```python
from build123d import *

# Parameters (mm, degrees)
BOSS_EXTRUDE1_DEPTH = 6


with BuildPart() as part:
    # Sketch1 → Boss-Extrude1 (new body)
    with BuildSketch(Plane.XY.offset(6)):
        Polygon((302.766666667, 244), (302.766666667, 250), (282.033333333, 250), (282.033333333, 244), (260.3, 244), (260.3, 250), (239.566666667, 250), (239.566666667, 244), (217.833333333, 244), (217.833333333, 250), (197.1, 250), (197.1, 244), (175.366666667, 244), (175.366666667, 250), (154.633333333, 250), (154.633333333, 244), (132.9, 244), (132.9, 250), (112.166666667, 250), (112.166666667, 244), (90.433333333, 244), (90.433333333, 250), (69.7, 250), (69.7, 244), (47.966666667, 244), (47.966666667, 250), (27.233333333, 250), (27.233333333, 244), (6, 244), (6, 227.227272727), (0, 227.227272727), (0, 204.954545455), (6, 204.954545455), (6, 181.681818182), (0, 181.681818182), (0, 159.409090909), (6, 159.409090909), (6, 136.136363636), (0, 136.136363636), (0, 113.863636364), (6, 113.863636364), (6, 90.590909091), (0, 90.590909091), (0, 68.318181818), (6, 68.318181818), (6, 45.045454545), (0, 45.045454545), (0, 22.772727273), (6, 22.772727273), (6, 6), (27.233333333, 6), (27.233333333, 0), (47.966666667, 0), (47.966666667, 6), (69.7, 6), (69.7, 0), (90.433333333, 0), (90.433333333, 6), (112.166666667, 6), (112.166666667, 0), (132.9, 0), (132.9, 6), (154.633333333, 6), (154.633333333, 0), (175.366666667, 0), (175.366666667, 6), (197.1, 6), (197.1, 0), (217.833333333, 0), (217.833333333, 6), (239.566666667, 6), (239.566666667, 0), (260.3, 0), (260.3, 6), (282.033333333, 6), (282.033333333, 0), (302.766666667, 0), (302.766666667, 6), (324, 6), (324, 22.772727273), (330, 22.772727273), (330, 45.045454545), (324, 45.045454545), (324, 68.318181818), (330, 68.318181818), (330, 90.590909091), (324, 90.590909091), (324, 113.863636364), (330, 113.863636364), (330, 136.136363636), (324, 136.136363636), (324, 159.409090909), (330, 159.409090909), (330, 181.681818182), (324, 181.681818182), (324, 204.954545455), (330, 204.954545455), (330, 227.227272727), (324, 227.227272727), (324, 244), align=None)
    extrude(amount=-BOSS_EXTRUDE1_DEPTH)


solid = part.part
```
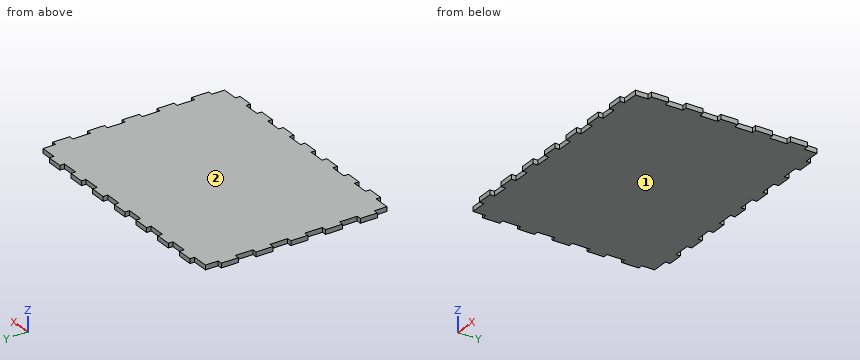
Part model, mm, in its own coordinate system. Face numbers are marked on the shaded views. Coordinates: 2 decimals unless noted, no trailing zeros. Loops run counter-clockwise (first coordinate to the right, second up) from the corner with the lowest first, then second, coordinate; pieces in that order, holes last. Notation, with made-up numbers: (7.25, -24.5) - (45.25, -24.5) arc R12 ccw to (45.25, -3.5) - close; hole circle Ø11 at (-32, -11). An arc over 180 degrees is marked (long way). Write item = value, one per line. Start each with the question number.
Item 1: Cut at A-A, the plane x = 184.5. Give the cut face in (y, z).
Item 2: Cut at B-B, the plane y = 200. Give the cut face in (x, z), and give its area (3 significant figures).
Item 3: Flat gauge pins, fed straight in: pin 1 Ø1.8 at (x, z) = (4, 4) entering from -Y; pin 2 Ø1.8 at (y, z) = (1.5, 2.5) entering from +X; pin 3 Ø1.8 at (x, z) = (3, 3.5) entering from +Y. Where does each tip first touch, or does it go through?
Item 4: Wall check: L1, parallel to X at y = 194, z = 3.75; L2, parallel to Y at x = 274, z = 1. Give the ranges that are in metal, low to high. Write a range as from..to.
Item 5: Mould opens along Z. For the marked faces 1 and 2 say: released by +Z, released by -Z, zero draft, split by the parting line, or undercut.
The answers:
q1.outline = (6, 0) - (244, 0) - (244, 6) - (6, 6) - close
q2.outline = (6, 0) - (324, 0) - (324, 6) - (6, 6) - close
q2.area = 1,910 mm2
q3.pin_1 = 22.77
q3.pin_2 = 302.77
q3.pin_3 = 227.23
q4.L1 = 6..324
q4.L2 = 6..244
q5.face_1 = released by -Z
q5.face_2 = released by +Z
